The listing builds one solid part. Answer for the finished solid, in the listing's coordinates (mm). Face numbers are marked on the shaded views. Coordinates: 2 decimals unless noted, no trailing zeros. Write each loop counter-clockwise with the first axis right and the second up, starting at its lowest first coordinate (ties: lowest second). Pieces come first, ordered by that corner, then holes.
from build123d import *

# Parameters (mm, degrees)
BOSS_EXTRUDE1_DEPTH = 48.3616
FILLET1_R           = 3.3782
SKETCH2_R           = 1.905
CUT_EXTRUDE1_DEPTH  = 16.3416
SKETCH3_W           = 7.86892
SKETCH3_H           = 7.86892
SKETCH3_R           = 1.35255
BOSS_EXTRUDE2_DEPTH = 0.762
SKETCH4_W           = 12.7
SKETCH4_H           = 5.588
SKETCH4_W_2         = 8.636
SKETCH4_H_2         = 2.794
BOSS_EXTRUDE3_DEPTH = 9.906
SKETCH5_W           = 0.635
SKETCH5_H           = 0.635
BOSS_EXTRUDE4_DEPTH = 4.6736


with BuildPart() as part:
    # Sketch1 → Boss-Extrude1 (new body)
    with BuildSketch(Plane.XY):
        Polygon((0, 0), (67.51574, 0), (67.51574, 15.3416), (53.59908, 15.3416), (53.59908, 26.6446), (13.91666, 26.6446), (13.91666, 15.3416), (0, 15.3416), align=None)
    extrude(amount=-BOSS_EXTRUDE1_DEPTH)

    # Fillet1
    fillet1_edges = [part.edges().sort_by_distance(p)[0] for p in [
        (67.51574, 7.6708, -48.3616),
        (0, 7.6708, 0),
        (0, 7.6708, -48.3616),
        (67.51574, 7.6708, 0),
    ]]
    fillet(fillet1_edges, radius=FILLET1_R)

    # Sketch2 → Cut-Extrude1 (cut, through all)
    with BuildSketch(Plane(origin=(0, 15.3416, 0), x_dir=(1, 0, 0), z_dir=(0, 1, 0))):
        with Locations((3.3782, 3.3782)):
            Circle(SKETCH2_R)
        with Locations((64.13754, 44.9834)):
            Circle(SKETCH2_R)
    extrude(amount=-CUT_EXTRUDE1_DEPTH, mode=Mode.SUBTRACT)

    # Sketch3 → Boss-Extrude2 (add)
    with BuildSketch(Plane(origin=(0, 15.3416, 0), x_dir=(1, 0, 0), z_dir=(0, 1, 0))):
        with Locations((60.06592, 25.88768)):
            Rectangle(SKETCH3_W, SKETCH3_H)
        with Locations((60.06592, 25.88768)):
            Circle(SKETCH3_R, mode=Mode.SUBTRACT)
        with Locations((7.44982, 37.31768)):
            Rectangle(SKETCH3_W, SKETCH3_H)
        with Locations((7.44982, 37.31768)):
            Circle(SKETCH3_R, mode=Mode.SUBTRACT)
        with Locations((7.44982, 25.88768)):
            Rectangle(SKETCH3_W, SKETCH3_H)
        with Locations((7.44982, 25.88768)):
            Circle(SKETCH3_R, mode=Mode.SUBTRACT)
        with Locations((60.06592, 37.31768)):
            Rectangle(SKETCH3_W, SKETCH3_H)
        with Locations((60.06592, 37.31768)):
            Circle(SKETCH3_R, mode=Mode.SUBTRACT)
    extrude(amount=BOSS_EXTRUDE2_DEPTH)

    # Sketch4 → Boss-Extrude3 (add)
    with BuildSketch(Plane(origin=(0, 15.3416, 0), x_dir=(1, 0, 0), z_dir=(0, 1, 0))):
        with Locations((6.35, 17.88922)):
            Rectangle(SKETCH4_W, SKETCH4_H)
        with Locations((6.35, 17.88922)):
            Rectangle(SKETCH4_W_2, SKETCH4_H_2, mode=Mode.SUBTRACT)
    extrude(amount=BOSS_EXTRUDE3_DEPTH)

    # Sketch5 → Boss-Extrude4 (add)
    with BuildSketch(Plane(origin=(0, 15.3416, 0), x_dir=(1, 0, 0), z_dir=(0, 1, 0))):
        with Locations((55.79618, 16.52016)):
            Rectangle(SKETCH5_W, SKETCH5_H)
        with Locations((55.79618, 13.98016)):
            Rectangle(SKETCH5_W, SKETCH5_H)
        with Locations((55.79618, 11.44016)):
            Rectangle(SKETCH5_W, SKETCH5_H)
    extrude(amount=BOSS_EXTRUDE4_DEPTH)


solid = part.part
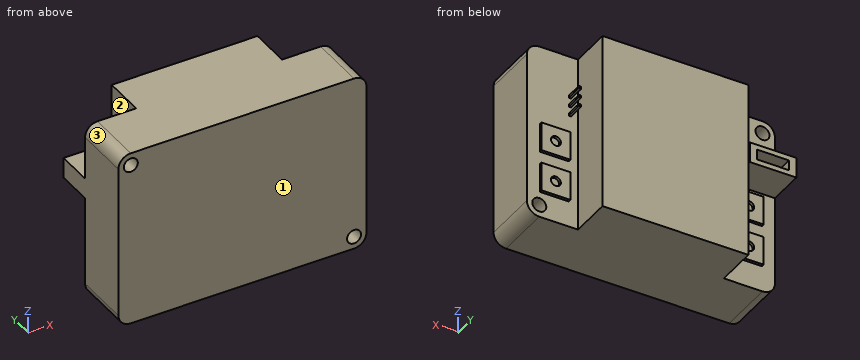
Q1. The part is cut by section A-A, the plane y = 19.25. Write down the section's boundary in (x, z).
Answers below:
outline: (0, -20.68) - (12.7, -20.68) - (12.7, -15.1) - (0, -15.1) - close; (13.92, -48.36) - (53.6, -48.36) - (53.6, 0) - (13.92, 0) - close; (55.48, -16.84) - (56.11, -16.84) - (56.11, -16.2) - (55.48, -16.2) - close; (55.48, -14.3) - (56.11, -14.3) - (56.11, -13.66) - (55.48, -13.66) - close; (55.48, -11.76) - (56.11, -11.76) - (56.11, -11.12) - (55.48, -11.12) - close; hole (2.03, -19.29) - (10.67, -19.29) - (10.67, -16.49) - (2.03, -16.49) - close
Q2. The part is cut by section C-C, the plane z = -9. Write down the section's boundary in (x, y).
Answers below:
outline: (0, 0) - (67.52, 0) - (67.52, 15.34) - (53.6, 15.34) - (53.6, 26.64) - (13.92, 26.64) - (13.92, 15.34) - (0, 15.34) - close
Q3. The part is cut by section D-D, the plane x = 7. Write down the section's boundary in (y, z).
Answers below:
outline: (0, -48.36) - (15.34, -48.36) - (15.34, -41.25) - (16.1, -41.25) - (16.1, -38.59) - (15.34, -38.59) - (15.34, -36.04) - (16.1, -36.04) - (16.1, -33.38) - (15.34, -33.38) - (15.34, -29.82) - (16.1, -29.82) - (16.1, -27.16) - (15.34, -27.16) - (15.34, -24.61) - (16.1, -24.61) - (16.1, -21.95) - (15.34, -21.95) - (15.34, -20.68) - (25.25, -20.68) - (25.25, -19.29) - (15.34, -19.29) - (15.34, -16.49) - (25.25, -16.49) - (25.25, -15.1) - (15.34, -15.1) - (15.34, 0) - (0, 0) - close
Q4. Given pin 1 (2.5 mm diameter, centred on x = 60, z = -27, fed in from +Y); pin 2 (3.5 mm diameter, centred on x = 64.14, z = -44.98, fed in from +Y) (1 decimal); pin 3 (0.8 mm diameter, centred on x = 60.5, z = -37, fed in from +Y); pin 4 (3 mm diameter, centred on x = 9.5, z = -19, fed in from +Y), each flat-ended and moving along its own axis, determine where each tip first touches the part or whether it passes through.
Answers below:
pin 1: stops at y = 16.1
pin 2: passes through
pin 3: stops at y = 15.34
pin 4: stops at y = 25.25
Q5. Find the intervals of material crossed by probe 1 along X at (y, z) = (23.25, -18); probe 2 along X at (y, z) = (4.5, -45); probe 3 along X at (y, z) = (16, -20.5), in increasing order.
Answers below:
probe 1: x = 0 to 2.03, 10.67 to 12.7, 13.92 to 53.6
probe 2: x = 0 to 62.23, 66.04 to 67.52
probe 3: x = 0 to 12.7, 13.92 to 53.6
Q6. Determine the mould class of the marked faces 1, 2 and 3 for opening direction X: released by +X, released by -X, zero draft, split by the parting line, or undercut.
Answers below:
face 1: zero draft
face 2: undercut
face 3: released by -X
Q7. The part is cut by section B-B, the plane y = 24.25. Write down the section's boundary in (x, z), then the cut area to 3 significant figures.
Answers below:
outline: (0, -20.68) - (12.7, -20.68) - (12.7, -15.1) - (0, -15.1) - close; (13.92, -48.36) - (53.6, -48.36) - (53.6, 0) - (13.92, 0) - close; hole (2.03, -19.29) - (10.67, -19.29) - (10.67, -16.49) - (2.03, -16.49) - close
area: 1,970 mm2
